Design review of the part built by this model. Coordinates are the model's own, in mm. A direction names the side the tool comes from. Coordinates: 2 decimals unless noted, no trailing zeros. Loops run counter-clockwise (first coordinate to the right, second up) from the corner with the lowest first, then second, coordinate; pieces in that order, holes last. Notation, with made-up numbers: (-2, -10) -> (32, -10) arc R9 ccw to (32, -1) -> close; hole circle Ø9 at (42.5, 2). An arc over 180 degrees is marked (long way). Answer in a Markdown table with one row per item.
```python
from build123d import *


with BuildPart() as part:
    # Croquis1 → Revolución1 (revolve)
    with BuildSketch(Plane.XY, mode=Mode.PRIVATE) as revoluci_n1_sk:
        Polygon((0, 0), (0, 1000), (0, 1050.939325751), (0, 1179.596825217), (33.678420865, 1179.596825217), (33.678420865, 1154.729022207), (21.987750201, 1154.729022207), (21.987750201, 1050.939325751), (102.820969977, 1050.939325751), (102.820969977, 1025.469662875), (50, 1025.469662875), (50, 1000), (142.43669746, 976.989967783), (50, 921.400938378), (148.786291167, 896.810317934), (50, 837.402807764), (148.786291167, 812.812187319), (50, 753.404677149), (148.786291167, 728.814056705), (50, 669.406546534), (148.786291167, 644.81592609), (50, 585.40841592), (148.786291167, 560.817795475), (50, 501.410285305), (148.786291167, 476.819664861), (50, 417.41215469), (148.786291167, 392.821534246), (50, 333.414024076), (148.786291167, 308.823403631), (50, 249.415893461), (148.786291167, 224.825273017), (50, 165.417762846), (50, 0), align=None)
    revolve(revoluci_n1_sk.sketch.rotate(Axis((0, 0, 0), (0, 1, 0)), 90), axis=Axis((0, 0, 0), (0, 1, 0)))


solid = part.part
```
(1) Draft analysis for pull direction Y (two halves, no side actions). For faces 1 (the cylindrical face through (-28.4, 1167, -18.1)), 2 (the flat face through (-1, 0, 1)), 3 (the conical face through (49.84, 583.87, -25.92)), state which applies: pulls with the +Y half, pulls with the -Y half, needs draft (parallel to the pull), parting line crosses it, or undercut.
Evaluation:
| item | result |
|---|---|
| face 1 | needs draft |
| face 2 | pulls with the -Y half |
| face 3 | undercut |
(2) To check wall thickness, follow probe 1 along X at (y, z) = (126.5, -37); probe 2 along Y at (x, z) = (25, -40); probe 3 along X at (y, z) = (810, -23). State the ranges of each line that lie inside material, in increasing order.
Evaluation:
| item | result |
|---|---|
| probe 1 | x = -33.63 to 33.63 |
| probe 2 | y = 0 to 1050.94 |
| probe 3 | x = -142.26 to 142.26 |
(3) Take a section at C-C on y = 133.5. Give the boundary of the cut face in (x, z), and give its area (3 significant figures).
Evaluation:
| item | result |
|---|---|
| outline | circle Ø100 at (0, 0) |
| area | 7,850 mm² |
(4) Take a section at A-A on x = 131. Count the separate pieces of the cut face and the enclosed holes in it, and give its area (3 significant figures).
Evaluation:
| item | result |
|---|---|
| separate pieces | 10 |
| enclosed holes | 0 |
| area | 13,400 mm² |
(5) Tool access review of faces 4 (the conical face through (-16.46, 840.29, -52.27)), 5 (the cylindrical face through (-15.02, 81.55, -47.69)): name each direction out of +Z, -Z, +X, -X, +Y, -Y from which nothing blocks a thin tool from reaching the whole face with its end or side.
Evaluation:
| item | result |
|---|---|
| face 4 | none |
| face 5 | -Y |
(6) For pin 1 (4 mm diameter, centred on x = 99, z = 89, fed in from -Y); pin 2 (5 mm diameter, centred on x = -15, z = -87, fed in from -Y); pin 3 (4 mm diameter, centred on x = -18, z = 99.5, fed in from -Y), all flat-tipped, find the tip position at first contact; note any pin that passes through.
Evaluation:
| item | result |
|---|---|
| pin 1 | stops at y = 214.2 |
| pin 2 | stops at y = 186.94 |
| pin 3 | stops at y = 194.95 |
